Here's the drawing with two shaded views (mm, measured from the low corner). I have some questions. Round coordinates to 2 decimals unless told otherwise and drop trailing zeros. Loops run counter-clockwise (first coordinate to the right, second up) from the corner with the lowest first, then second, coordinate; pieces in that order, holes last. Notation, with made-up numbers: (61, 14.5) -> (117, 14.5) arc R16 ccw to (117, 42.5) -> close; hole circle Ø1 at (-36, -5.75). An arc over 180 degrees is marked (long way). Write each question's results on one line, items separated by ' | '. Start each with the question number.
1) Imagine slicing it at A-A, the plane z = 13. List the corners of the cut face in (x, y) for me.
2) If I drill on probe 1 along X at (y, z) = (0.5, 14); probe 2 along X at (y, z) = (4.5, 20.5); probe 3 along X at (y, z) = (3.75, 53.5), over which ranges is the centre line in solid material (lowest first)?
3) Imagine slicing it at B-B, the plane y = 4.5. Give the number of separate pieces and of enclosed holes in the cut face, plus the area to 3 significant figures.
4) For P1, Ø0.5, axis at x = 0.5, y = 4, coming from the -Z side; P2, Ø1.5, axis at y = 1, z = 24.5, coming from the -X side; P3, Ø3, axis at y = 1.5, z = 25.5, coming from the +X side, each with a flat end and sliding along its axis, tell me the tip position at first contact or that it passes through.
5) We'd pull the mould along X, two halves only. Please class the marked faces 1, 2 and 3: pulls with the +X half, pulls with the -X half, needs draft (parallel to the pull), parting line crosses it, or undercut.
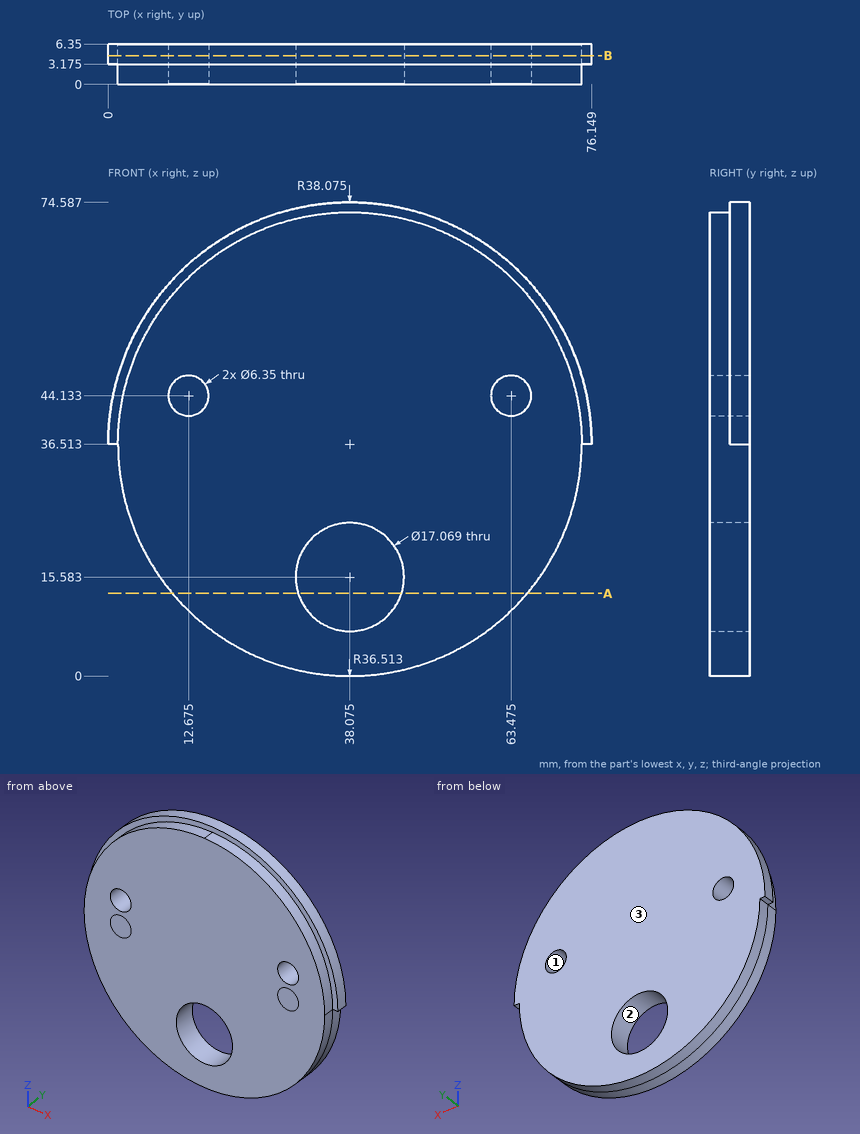
Checked values:
1) outline: (10.14, 0) -> (29.94, 0) -> (29.94, 6.35) -> (10.14, 6.35) -> close; (46.21, 0) -> (66.01, 0) -> (66.01, 6.35) -> (46.21, 6.35) -> close
2) probe 1: 9.33 to 29.69, 46.46 to 66.82 | probe 2: 5.26 to 31.1, 45.05 to 70.89 | probe 3: 4 to 72.15
3) separate pieces: 1 | enclosed holes: 3 | area: 4,080 mm^2
4) P1: z = 36.51 | P2: x = 3.34 | P3: x = 73.33
5) face 1: undercut | face 2: undercut | face 3: needs draft
